```python
from build123d import *

# Parameters (mm, degrees)
F0_W      = 92.131638
F0_H      = 77.216
F1_DEPTH  = 13.97
F3_DEPTH  = 13.971
F5_DEPTH  = 38.609
F6_DEPTH  = 38.609
F8_DEPTH  = 3.81
F9_R      = 2.54
F10_DEPTH = 25.4
F12_DEPTH = 3.175


with BuildPart() as f1:
    # F0 (on Top) → F1 (new body)
    with BuildSketch(Plane.XY):
        Rectangle(F0_W, F0_H)
    extrude(amount=F1_DEPTH)

    # F2 (on face) → F3 (intersect, through all)
    with BuildSketch(Plane.XY.offset(13.97)):
        with BuildLine():
            Line((46.065819, 0), (46.065819, 21.59))
            ThreePointArc((46.065819, 21.59), (0, 38.608), (-46.065819, 21.59))
            Line((-46.065819, 21.59), (-46.065819, 0))
            Line((-46.065819, 0), (-46.065819, -21.59))
            ThreePointArc((-46.065819, -21.59), (0, -38.608), (46.065819, -21.59))
            Line((46.065819, -21.59), (46.065819, 0))
        make_face()
    extrude(amount=-F3_DEPTH, mode=Mode.INTERSECT)

    # F4 (on Front) → F5 (cut, through all)
    with BuildSketch(Plane.XZ):
        Polygon((30.571819, 13.97), (30.571819, 12.7), (30.571819, 11.43), (42.001819, 11.43), (42.001819, 13.97), align=None)
        Polygon((19.095909, 13.97), (19.095909, 12.7), (19.095909, 11.43), (27.985909, 11.43), (27.985909, 12.7), (27.985909, 13.97), align=None)
        Polygon((-16.51, 13.97), (-16.51, 12.7), (-16.51, 11.43), (0, 11.43), (16.51, 11.43), (16.51, 12.7), (16.51, 13.97), align=None)
        Polygon((-27.985909, 13.97), (-27.985909, 12.7), (-27.985909, 11.43), (-19.095909, 11.43), (-19.095909, 12.7), (-19.095909, 13.97), align=None)
        Polygon((-30.571819, 13.97), (-42.001819, 13.97), (-42.001819, 11.43), (-30.571819, 11.43), (-30.571819, 12.7), align=None)
    extrude(amount=-F5_DEPTH, mode=Mode.SUBTRACT)

    # F4 (on Front) → F6 (cut, through all)
    with BuildSketch(Plane.XZ):
        Polygon((30.571819, 13.97), (30.571819, 12.7), (30.571819, 11.43), (42.001819, 11.43), (42.001819, 13.97), align=None)
        Polygon((19.095909, 13.97), (19.095909, 12.7), (19.095909, 11.43), (27.985909, 11.43), (27.985909, 12.7), (27.985909, 13.97), align=None)
        Polygon((-16.51, 13.97), (-16.51, 12.7), (-16.51, 11.43), (0, 11.43), (16.51, 11.43), (16.51, 12.7), (16.51, 13.97), align=None)
        Polygon((-27.985909, 13.97), (-27.985909, 12.7), (-27.985909, 11.43), (-19.095909, 11.43), (-19.095909, 12.7), (-19.095909, 13.97), align=None)
        Polygon((-30.571819, 13.97), (-42.001819, 13.97), (-42.001819, 11.43), (-30.571819, 11.43), (-30.571819, 12.7), align=None)
    extrude(amount=F6_DEPTH, mode=Mode.SUBTRACT)

    # F7 (on face) → F8 (cut)
    with BuildSketch(Plane(origin=(0, 0, 0), x_dir=(1, 0, 0), z_dir=(0, 0, -1))):
        with BuildLine():
            ThreePointArc((-15.552723, 4.8514), (-18.983181, 3.430458), (-20.404123, 0))
            ThreePointArc((-20.404123, 0), (-18.983181, -3.430458), (-15.552723, -4.8514))
            Line((-15.552723, -4.8514), (-11.483329, -9.3218))
            Line((-11.483329, -9.3218), (-11.483329, -13.1318))
            Line((-11.483329, -13.1318), (-9.197329, -13.1318))
            ThreePointArc((-9.197329, -13.1318), (-0.624908, -16.856695), (5.107457, -9.4742))
            Line((5.107457, -9.4742), (5.107457, -6.0325))
            Line((5.107457, -6.0325), (15.572257, -6.0325))
            Line((15.572257, -6.0325), (15.572257, 0))
            Line((15.572257, 0), (15.572257, 6.0325))
            Line((15.572257, 6.0325), (5.107457, 6.0325))
            Line((5.107457, 6.0325), (5.107457, 9.4742))
            ThreePointArc((5.107457, 9.4742), (-0.624908, 16.856695), (-9.197329, 13.1318))
            Line((-9.197329, 13.1318), (-11.483329, 13.1318))
            Line((-11.483329, 13.1318), (-11.483329, 9.3218))
            Line((-11.483329, 9.3218), (-15.552723, 4.8514))
        make_face()
    extrude(amount=-F8_DEPTH, mode=Mode.SUBTRACT)

    # F9 (on face) → F10 (cut)
    with BuildSketch(Plane(origin=(0, 0, 3.81), x_dir=(1, 0, 0), z_dir=(0, 0, -1))):
        with Locations((-2.512543, -7.0104)):
            Circle(F9_R)
        with Locations((-2.512543, 7.0104)):
            Circle(F9_R)
    extrude(amount=-F10_DEPTH, mode=Mode.SUBTRACT)

    # F11 (on face) → F12 (cut)
    with BuildSketch(Plane.XY.offset(11.43)):
        Polygon((-5.18885, -2.3749), (-7.865157, -7.0104), (-5.18885, -11.6459), (0.163764, -11.6459), (2.840071, -7.0104), (0.163764, -2.3749), align=None)
        Polygon((0.163764, 11.6459), (-5.18885, 11.6459), (-7.865157, 7.0104), (-5.18885, 2.3749), (0.163764, 2.3749), (2.840071, 7.0104), align=None)
    extrude(amount=-F12_DEPTH, mode=Mode.SUBTRACT)


solid = f1.part
```
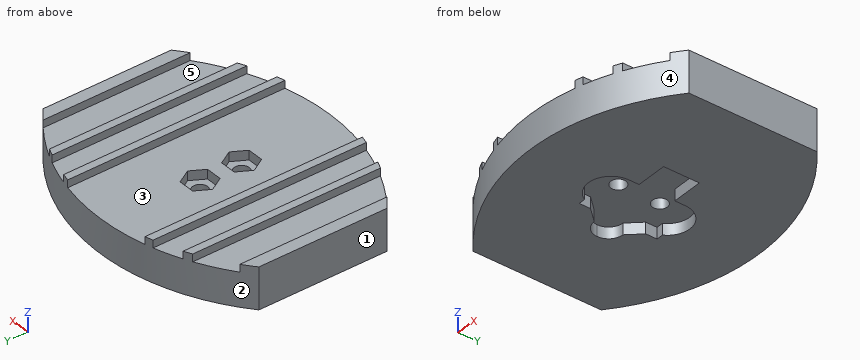
Work out the finished part from the listing and answer in its coordinate system (mm). Face numbers are marked on the shaded views. A direction names the side the tool comes from. Coordinates: 2 decimals unless noted, no trailing zeros. Loops run counter-clockwise (first coordinate to the right, second up) from the corner with the lowest first, then second, coordinate; pieces in that order, holes last. Notation, with made-up numbers: (8, -16.75) - (62, -16.75) arc R16 cw to (62, 11.25) - close; hole circle Ø9 at (6.5, 71.25). An arc over 180 degrees is marked (long way). Use a Markdown table: item, result.
Item 1: Find section D-D, the plane x = -21.5. Determine the outline of the cut face in (y, z), and give its area (3 significant figures).
Evaluation:
| item | result |
|---|---|
| outline | (-35.27, 0) - (35.27, 0) - (35.27, 11.43) - (-35.27, 11.43) - close |
| area | 806 mm2 |
Item 2: Find section A-A, the plane y = -19.5. Determine the outline of the cut face in (x, z), and give its area (3 significant figures).
Evaluation:
| item | result |
|---|---|
| outline | (-46.07, 0) - (46.07, 0) - (46.07, 13.97) - (42, 13.97) - (42, 11.43) - (30.57, 11.43) - (30.57, 13.97) - (27.99, 13.97) - (27.99, 11.43) - (19.1, 11.43) - (19.1, 13.97) - (16.51, 13.97) - (16.51, 11.43) - (-16.51, 11.43) - (-16.51, 13.97) - (-19.1, 13.97) - (-19.1, 11.43) - (-27.99, 11.43) - (-27.99, 13.97) - (-30.57, 13.97) - (-30.57, 11.43) - (-42, 11.43) - (-42, 13.97) - (-46.07, 13.97) - close |
| area | 1,100 mm2 |
Item 3: Consider probe 1 along X at (y, z) = (-12, 11.75); probe 2 along Z at (x, y) = (2, -31.5); probe 3 along Y at (x, z) = (7, 2.25). Determine where each line is inside the solid, lowest interval first. Write a range as from..to.
Evaluation:
| item | result |
|---|---|
| probe 1 | x = -46.07..-42, -30.57..-27.99, -19.1..-16.51, 16.51..19.1, 27.99..30.57, 42..46.07 |
| probe 2 | z = 0..11.43 |
| probe 3 | y = -38.26..-6.03, 6.03..38.26 |
Item 4: The mould has two halves that part along X. Classify the marked faces 1, 2 and 3: +X half, -X half, draft (parallel to the pull), parting line (faces both ways), or undercut.
Evaluation:
| item | result |
|---|---|
| face 1 | -X half |
| face 2 | parting line |
| face 3 | undercut |
Item 5: Given pin 1 Ø1.9 at (x, z) = (10.5, 2) entering from -Y; pin 2 Ø0.7 at (x, z) = (-10.5, 2.5) entering from -Y; pin 3 Ø3 at (x, y) = (-0.5, -18) entering from -Z; pin 4 Ø1 at (y, z) = (25, 11) entering from -X, each flat-ended and moving along its own axis, determine where each tip first touches the part or whether it passes through.
Evaluation:
| item | result |
|---|---|
| pin 1 | stops at y = -37.96 |
| pin 2 | stops at y = -37.88 |
| pin 3 | stops at z = 0 |
| pin 4 | stops at x = -42.43 |
Item 6: For the marked faces 4 and 5, determine the directions among +Z, -Z, +X, -X, +Y, -Y from which every point of the face is accessible in a straight line to the end or side of a thin tool.
Evaluation:
| item | result |
|---|---|
| face 4 | +Z, -Z, -Y |
| face 5 | +Z, +Y, -Y |
Item 7: Find section B-B, the plane x = 11.5. Determine the outline of the cut face in (y, z), and give its area (3 significant figures).
Evaluation:
| item | result |
|---|---|
| outline | (-37.67, 0) - (-6.03, 0) - (-6.03, 3.81) - (6.03, 3.81) - (6.03, 0) - (37.67, 0) - (37.67, 11.43) - (-37.67, 11.43) - close |
| area | 815 mm2 |
Item 8: Find section C-C, the plane y = 23. Determine the outline of the cut face in (x, z).
Evaluation:
| item | result |
|---|---|
| outline | (-44.36, 0) - (44.36, 0) - (44.36, 13.97) - (42, 13.97) - (42, 11.43) - (30.57, 11.43) - (30.57, 13.97) - (27.99, 13.97) - (27.99, 11.43) - (19.1, 11.43) - (19.1, 13.97) - (16.51, 13.97) - (16.51, 11.43) - (-16.51, 11.43) - (-16.51, 13.97) - (-19.1, 13.97) - (-19.1, 11.43) - (-27.99, 11.43) - (-27.99, 13.97) - (-30.57, 13.97) - (-30.57, 11.43) - (-42, 11.43) - (-42, 13.97) - (-44.36, 13.97) - close |
